Could you check a few things on this drawing? It's one solid part, dimensions in mm from its lowest x, y, z. A direction names the side the tool comes from. Coordinates: 2 decimals unless noted, no trailing zeros. Loops run counter-clockwise (first coordinate to the right, second up) from the corner with the lowest first, then second, coordinate; pieces in that order, holes last. Notation, with made-up numbers: M -9.5,-2 L 11.5,-2 A12 ccw 11.5,5 Z; hole C 23,-23.75 d7. An arc over 180 degrees is marked long. Answer as a JSON object with one key per item and string values. Group by question number.
Item 1: Suppose I cut it at D-D (x = 8.5). Write out the boundary of the cut face in (y, z) (3 decimals), then the cut area to 3 significant figures.
Item 2: We'd pull the mould along Y, two halves only. Please class the marked faces 4, 5, 6 and 7: +Y half, -Y half, draft (parallel to the pull), parting line (faces both ways), or undercut.
Item 3: Suppose I cut it at A-A (z = 7). Write out the boundary of the cut face in (x, y) (3 decimals).
Item 4: Suppose I cut it at C-C (z = 4.25). Write out the boundary of the cut face in (x, y) (3 decimals).
Item 5: If I drill on line 1 (Y direction, x = 15, z = 3.5) (3 decimals); line 2 (X direction, y = 14.5, z = 2.75); line 3 (Z direction, x = 9.5, y = 6.75), over which ranges is the centre line in solid material (lowest first)?
Item 6: Which directions (+Z, -Z, +X, -X, +Y, -Y) give clear straight access to the entire face, cutting with the end or side of a thin tool? Please do the marked faces 1, 2 and 3.
Item 7: Suppose I cut it at B-B (x = 11.43). Write out the boundary of the cut face in (y, z) (3 decimals).
Item 8: I'm going to push flat-ended pins straight in: pin 1 Ø4.5 at (x, y) = (12.5, 11) entering from -Z; pin 2 Ø1.5 at (x, z) = (15.5, 5.5) entering from -Y (3 decimals); pin 3 Ø1.9 at (x, z) = (12.5, 4.5) entering from +Y (3 decimals); pin 4 Ø2 at (x, y) = (8, 3) entering from -Z. Where does each tip first touch, or does it pass through?
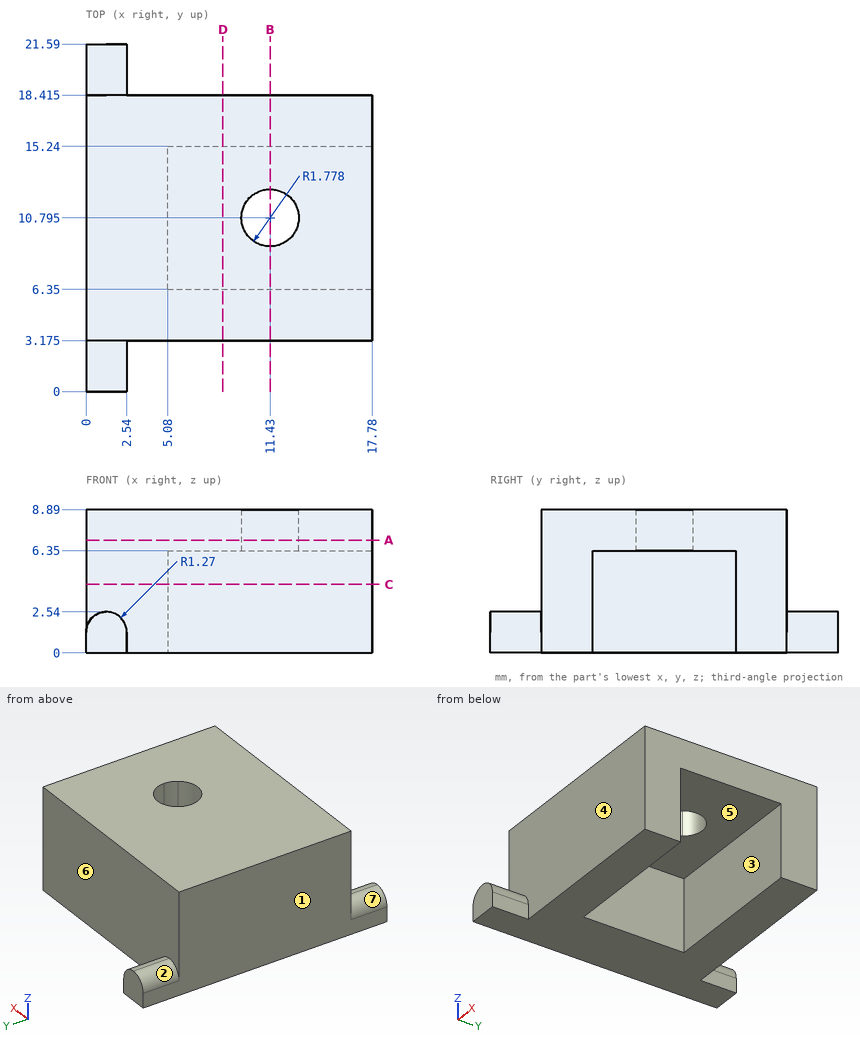
From the geometry:
{
 "1": {"outline": "M 3.175,0 L 6.35,0 L 6.35,6.35 L 15.24,6.35 L 15.24,0 L 18.415,0 L 18.415,8.89 L 3.175,8.89 Z", "area": "79.0 mm2"},
 "2": {"face 4": "-Y half", "face 5": "undercut", "face 6": "+Y half", "face 7": "draft"},
 "3": {"outline": "M 0,3.175 L 17.78,3.175 L 17.78,18.415 L 0,18.415 Z; hole C 11.43,10.795 d3.556"},
 "4": {"outline": "M 0,3.175 L 17.78,3.175 L 17.78,6.35 L 5.08,6.35 L 5.08,15.24 L 17.78,15.24 L 17.78,18.415 L 0,18.415 Z"},
 "5": {"line 1": "3.175 to 6.35, 15.24 to 18.415", "line 2": "0 to 5.08", "line 3": "6.35 to 8.89"},
 "6": {"face 1": "+Z, -Z, -X, +Y, -Y", "face 2": "+Z, -X, +Y", "face 3": "-Z, +X"},
 "7": {"outline": "M 3.175,0 L 6.35,0 L 6.35,6.35 L 9.017,6.35 L 9.017,8.89 L 3.175,8.89 Z; M 12.573,6.35 L 15.24,6.35 L 15.24,0 L 18.415,0 L 18.415,8.89 L 12.573,8.89 Z"},
 "8": {"pin 1": "z = 6.35", "pin 2": "y = 3.175", "pin 3": "y = 18.415", "pin 4": "z = 0"}
}
